Source: CAD feature listing. Evaluate the final solid. Frame: model axes, mm. A direction names the side the tool comes from. Give positions to 0.01 mm unless a question says otherwise; leave off trailing zeros. Write each loop counter-clockwise with the first axis right and the second up, starting at its lowest first coordinate (ties: lowest second). Pieces come first, ordered by that corner, then holes. Notation, with made-up numbers: M 36.5,85.5 L 95.5,85.5 A30 cw 95.5,107.5 Z; hole C -35.5,24.25 d3. An arc over 180 degrees is marked long. Return JSON: item names as keys, results as strings.
Autodesk Inventor part; units mm, degrees
ref_plane "YZ Plane" through (0, 0, 0) normal (1, 0, 0) x (0, 1, 0)
ref_plane "XZ Plane" through (0, 0, 0) normal (0, 1, 0) x (-1, 0, 0)
ref_plane "XY Plane" through (0, 0, 0) normal (0, 0, 1) x (1, 0, 0)
sketch "Sketch1" plane through (0, 0, 0) normal (0, 0, 1) x (1, 0, 0)
  line L0 (-12.1708, 16.0073) -> (13.2292, 16.0073)
  line L1 (13.2292, 16.0073) -> (13.2292, -34.7927)
  line L2 (13.2292, -34.7927) -> (-12.1708, -34.7927)
  line L3 (-12.1708, -34.7927) -> (-12.1708, 16.0073)
  line L4 (11.9592, 14.7373) -> (-10.9008, 14.7373)
  line L5 (-10.9008, 14.7373) -> (-10.9008, -33.5227)
  line L6 (-10.9008, -33.5227) -> (11.9592, -33.5227)
  line L7 (11.9592, -33.5227) -> (11.9592, 14.7373)
  point P0 (0, 0)
  dimension "d0" = 25.4
  dimension "d1" = 50.8
  dimension "d2" = 1.27
extrude "Extrusion1" add sketch "Sketch1" along normal blind 406.4
sketch "Sketch2" plane through (-12.1708, 16.0073, 0) normal (0, 1, 0) x (1, 0, 0)
  circle A0 centre (12.7, -12.7) radius 1.7272
  line L0 (25.4, 0) -> (0, 0)
  line L1 (0, 0) -> (0, -406.4)
  point P0 (12.1708, 0)
  dimension "d5" = 3.4544
  dimension "d6" = 12.7
  dimension "d7" = 12.7
extrude "Extrusion2" cut sketch "Sketch2" against normal through all
pattern_linear "Rectangular Pattern1" count 16 spacing 25.4 along (0, 0, 1) of "Extrusion2"
equation "\"d3\" = d13"
equation "\"d13\" = 406.4"
properties part number "VerseFrame 16in"
1) Cut plane C-C, the plane y = -7.5. Return the cut outline in (x, z), then the cut area to 3 significant figures.
Numbers:
{"outline": "M -12.17,0 L -10.9,0 L -10.9,406.4 L -12.17,406.4 Z; M 11.96,0 L 13.23,0 L 13.23,406.4 L 11.96,406.4 Z", "area": "1,030 mm²"}
2) Cut plane A-A, the plane x = 8.5. Return the cut outline in (y, z), then the cut area to 3 significant figures.
Numbers:
{"outline": "M -34.79,0 L -33.52,0 L -33.52,406.4 L -34.79,406.4 Z; M 14.74,0 L 16.01,0 L 16.01,406.4 L 14.74,406.4 Z", "area": "1,030 mm²"}
3) Set-up query: faces 1 (the face through (11.959, -10, 200)), 2 (the face through (-12, -9, 406.4)). Return all of +Z, -Z, +X, -X, +Y, -Y with unobstructed straight access to the full face (end or side cutting, diameter ignored); none if empty.
Numbers:
{"face 1": "+Z, -Z", "face 2": "+Z, +X, -X, +Y, -Y"}
4) Line query: line 1 (Y direction, x = -2.5, z = 311.5); line 2 (X direction, y = -7, z = 177); line 3 (X direction, y = -33.95, z = 38.1). Output: solid intervals per line, ascending. Write a range as [from, to].
Numbers:
{"line 1": "y = [-34.79, -33.52], [14.74, 16.01]", "line 2": "x = [-12.17, -10.9], [11.96, 13.23]", "line 3": "x = [-12.17, -1.2], [2.26, 13.23]"}
5) Draft query along Y for faces 3 (the face through (0, -33.523, 200)), 4 (the face through (0, 16.007, 200)), 5 (the face through (-12, -9, 0)). Return one class per face: released by +Y, released by -Y, zero draft, split by the parting line, or undercut.
Numbers:
{"face 3": "undercut", "face 4": "released by +Y", "face 5": "zero draft"}
6) Cut plane B-B, the plane z = 156. Return the cut outline in (x, y), then the cut area to 3 significant figures.
Numbers:
{"outline": "M -12.17,-34.79 L 13.23,-34.79 L 13.23,16.01 L -12.17,16.01 Z; hole M -10.9,-33.52 L 11.96,-33.52 L 11.96,14.74 L -10.9,14.74 Z", "area": "187 mm²"}
